Read the model definition and answer for the solid it produces. Units are mm, in the model's axes. Coordinates: 2 decimals unless noted, no trailing zeros. Order: outer loops, then holes, each group sorted by start corner. A loop starts at its lowest first (then second) coordinate and runs counter-clockwise, first axis right, second up. Notation, with made-up numbers: (-38.5, 83.25) -> (-29.5, 83.25) arc R25 ccw to (-29.5, 105.25) -> close; hole circle Ø2 at (22, 79.25). An arc over 180 degrees is marked (long way). Answer as a JSON object with one key per item and string values. Group by question number.
1) Determine the mould class of faces 1 (the cylindrical face through (-7.215, 0.105, 2.699)), 2 (the cylindrical face through (3.31, -1.67, 1.48)), 3 (the cylindrical face through (0.105, 7.215, 2.699)) for opening direction X: released by +X, released by -X, zero draft, split by the parting line, or undercut.
2) Consider L1, parallel to Y at x = 4, z = 2; L2, parallel to X at y = -4, z = 1.3; L3, parallel to X at y = -3.25, z = 2.6. Determine where each line is inside the solid, lowest interval first.
3) Section A-A on x = 4 is taken. Count the separate pieces of the cut face and the enclosed holes in it, and give its area (3 significant figures).
4) Section C-C on z = 0.7 is taken. Determine the outline of the cut face in (x, y), and give its area (3 significant figures).
from build123d import *

# Parameters (mm, degrees)
SKETCH1_W           = 15
SKETCH1_H           = 15
SKETCH1_R           = 1.5
BOSS_EXTRUDE1_DEPTH = 3
FILLET3_R           = 1
FILLET4_R           = 2


with BuildPart() as part:
    # Sketch1 → Boss-Extrude1 (new body)
    with BuildSketch(Plane.XY):
        Rectangle(SKETCH1_W, SKETCH1_H)
        with Locations((-4, 3)):
            Circle(SKETCH1_R, mode=Mode.SUBTRACT)
        with Locations((-4, -3)):
            Circle(SKETCH1_R, mode=Mode.SUBTRACT)
        with Locations(Location((4, -3, 0), (0, 0, 180))):
            Circle(SKETCH1_R, mode=Mode.SUBTRACT)
        with Locations(Location((4, 3, 0), (0, 0, 180))):
            Circle(SKETCH1_R, mode=Mode.SUBTRACT)
    extrude(amount=BOSS_EXTRUDE1_DEPTH)

    # Fillet3
    fillet3_edges = [part.edges().sort_by_distance(p)[0] for p in [
        (-7.5, 0, 3),
        (0, -7.5, 3),
        (7.5, 0, 3),
        (0, 7.5, 3),
    ]]
    fillet(fillet3_edges, radius=FILLET3_R)

    # Fillet4
    fillet4_edges = [part.edges().sort_by_distance(p)[0] for p in [
        (0, -7.5, 0),
        (-7.5, 0, 0),
        (7.5, 0, 0),
        (0, 7.5, 0),
    ]]
    fillet(fillet4_edges, radius=FILLET4_R - 0.0001)  # a hair under: the kernel refuses the full size


solid = part.part
Worked answers:
{
 "1": {"face 1": "released by -X", "face 2": "undercut", "face 3": "zero draft"},
 "2": {"L1": "y = -7.5 to -4.5, -1.5 to 1.5, 4.5 to 7.5", "L2": "x = -7.37 to -5.12, -2.88 to 2.88, 5.12 to 7.37", "L3": "x = -7.3 to -5.48, -2.52 to 2.52, 5.48 to 7.3"},
 "3": {"separate pieces": "3", "enclosed holes": "0", "area": "24.9 mm²"},
 "4": {"outline": "(-7.02, -7.02) -> (7.02, -7.02) -> (7.02, 7.02) -> (-7.02, 7.02) -> close; hole circle Ø3 at (-4, -3); hole circle Ø3 at (-4, 3); hole circle Ø3 at (4, -3); hole circle Ø3 at (4, 3)", "area": "169 mm²"}
}
